Geometry: see drawing. Coordinates: mm, zero at the bounding-box minimum. A direction names the side the tool comes from. Give positions to 0.01 mm unless a question says otherwise; leave off trailing zeros. Order: outer loops, then holes, each group sorted by start corner. A loop starts at its lowest first (then second) coordinate and runs counter-clockwise, first axis right, second up. Notation, with made-up numbers: M 83,-7.75 L 130,-7.75 A32 cw 130,18.25 Z; hole C 61,78.5 d5. An arc over 180 degrees is marked long. Use a Markdown table: item, result.
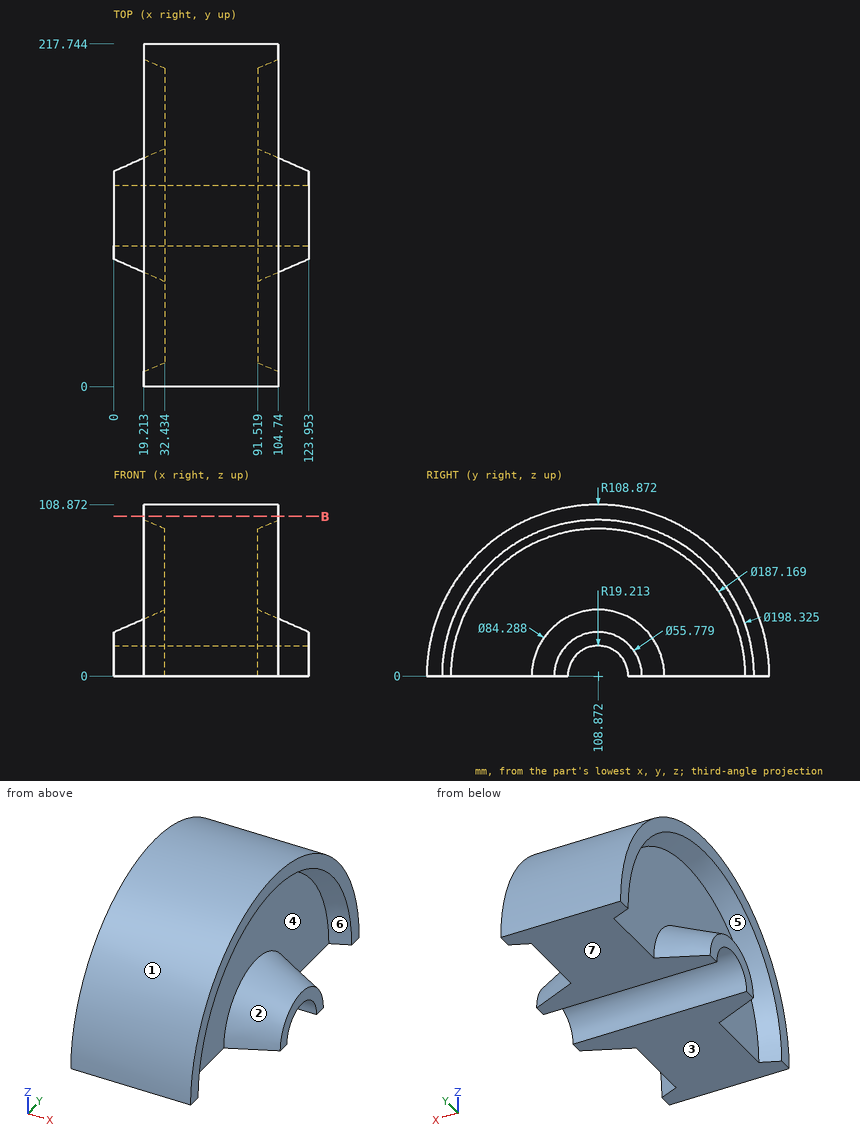
1) Cut plane B-B on z = 101.5. Return loops of the section in (x, y).
Response values:
| item | result |
|---|---|
| outline | M 19.21,69.49 L 104.74,69.49 L 104.74,148.25 L 19.21,148.25 Z |
2) Material intervals for line 1 (X direction, y = 46, z = 62) (1 decimal); line 2 (Z direction, x = 20.5, y = 129.5) (1 decimal); line 3 (X direction, y = 28, z = 72.5), sorted ascending. Write a range as from..to.
Response values:
| item | result |
|---|---|
| line 1 | x = 32.4..91.5 |
| line 2 | z = 0..30.6, 96.4..106.9 |
| line 3 | x = 19.21..104.74 |
3) Reachability of the marked faces 5, 6 and 7 from +Z, -Z, +X, -X, +Y, -Y: full face, straight path, thin tool, end or side. Return the list, or none.
Response values:
| item | result |
|---|---|
| face 5 | -X |
| face 6 | +X |
| face 7 | -Z, +X, -X, +Y, -Y |
4) First-contact query: pin 1 Ø1 at (x, y) = (32, 121.5) entering from -Z; pin 2 Ø3 at (x, y) = (104.5, 48.5) entering from -Z (1 decimal); pin 3 Ø1 at (y, z) = (71, 67.5) entering from +X. Flat tips, straight axial feed; report the tip coordinate or a pass-through.
Response values:
| item | result |
|---|---|
| pin 1 | stops at z = 14.03 |
| pin 2 | stops at z = 77.1 |
| pin 3 | stops at x = 91.52 |
5) Mould query, pull axis Y, two halves, no side actions, for the marked faces 1, 2, 3 and 4. Classes: released by +Y, released by -Y, zero draft, split by the parting line, or undercut.
Response values:
| item | result |
|---|---|
| face 1 | split by the parting line |
| face 2 | undercut |
| face 3 | zero draft |
| face 4 | undercut |
